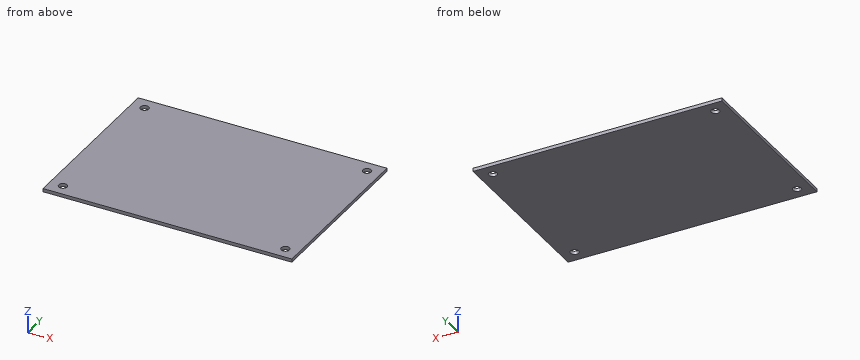
from build123d import *

# Parameters (mm, degrees)
SKETCH1_W           = 155
SKETCH1_H           = 110
BOSS_EXTRUDE1_DEPTH = 80
SKETCH2_W           = 151
SKETCH2_H           = 106
CUT_EXTRUDE1_DEPTH  = 78
SKETCH3_R           = 2.5
CUT_EXTRUDE2_DEPTH  = 2
SKETCH7_R           = 1.6
CUT_EXTRUDE7_DEPTH  = 2
SKETCH4_W           = 27.5
SKETCH4_H           = 46.8
CUT_EXTRUDE8_DEPTH  = 2
SKETCH8_W           = 4
SKETCH8_H           = 53
CUT_EXTRUDE9_DEPTH  = 2
SKETCH9_W           = 14
SKETCH9_H           = 14
CUT_EXTRUDE10_DEPTH = 2
SKETCH10_W          = 25.2
SKETCH10_H          = 71.2
SKETCH10_R          = 1.25
CUT_EXTRUDE12_DEPTH = 2
SKETCH11_R          = 2.5
SKETCH11_R_2        = 4.5
CUT_EXTRUDE13_DEPTH = 2
SKETCH12_W          = 151
SKETCH12_H          = 2
CUT_EXTRUDE14_DEPTH = 80


with BuildPart() as part:
    # Sketch1 → Boss-Extrude1 (new body)
    with BuildSketch(Plane.XY):
        with Locations((77.5, 55)):
            Rectangle(SKETCH1_W, SKETCH1_H)
    extrude(amount=BOSS_EXTRUDE1_DEPTH)

    # Sketch2 → Cut-Extrude1 (cut)
    with BuildSketch(Plane.XY.offset(80)):
        with Locations((77.5, 55)):
            Rectangle(SKETCH2_W, SKETCH2_H)
    extrude(amount=-CUT_EXTRUDE1_DEPTH, mode=Mode.SUBTRACT)

    # Sketch3 → Cut-Extrude2 (cut)
    with BuildSketch(Plane.XY.offset(2)):
        with Locations((145, 100.5)):
            Circle(SKETCH3_R)
        with Locations((145, 9.5)):
            Circle(SKETCH3_R)
        with Locations((10, 9.5)):
            Circle(SKETCH3_R)
        with Locations((10, 100.5)):
            Circle(SKETCH3_R)
    extrude(amount=-CUT_EXTRUDE2_DEPTH, mode=Mode.SUBTRACT)

    # Sketch7 → Cut-Extrude7 (cut)
    with BuildSketch(Plane(origin=(0, 110, 0), x_dir=(1, 0, 0), z_dir=(0, 1, 0))):
        with Locations((44.48, -20.14450396)):
            Circle(SKETCH7_R)
        with Locations((95.28, -17.14)):
            Circle(SKETCH7_R)
        with Locations((95.28, -62.86)):
            Circle(SKETCH7_R)
        with Locations((44.48, -47.62)):
            Circle(SKETCH7_R)
    extrude(amount=-CUT_EXTRUDE7_DEPTH, mode=Mode.SUBTRACT)

    # Sketch4 → Cut-Extrude8 (cut)
    with BuildSketch(Plane(origin=(155, 0, 0), x_dir=(0, 0, -1), z_dir=(1, 0, 0))):
        with Locations((-40, 82.5)):
            Rectangle(SKETCH4_W, SKETCH4_H)
    extrude(amount=-CUT_EXTRUDE8_DEPTH, mode=Mode.SUBTRACT)

    # Sketch8 → Cut-Extrude9 (cut)
    with BuildSketch(Plane(origin=(155, 0, 0), x_dir=(0, 0, -1), z_dir=(1, 0, 0))):
        with Locations((-68, 28.5)):
            Rectangle(SKETCH8_W, SKETCH8_H)
        with Locations((-76, 28.5)):
            Rectangle(SKETCH8_W, SKETCH8_H)
        with Locations((-60, 28.5)):
            Rectangle(SKETCH8_W, SKETCH8_H)
        with Locations((-52, 28.5)):
            Rectangle(SKETCH8_W, SKETCH8_H)
        with Locations((-44, 28.5)):
            Rectangle(SKETCH8_W, SKETCH8_H)
        with Locations((-36, 28.5)):
            Rectangle(SKETCH8_W, SKETCH8_H)
        with Locations((-28, 28.5)):
            Rectangle(SKETCH8_W, SKETCH8_H)
        with Locations((-20, 28.5)):
            Rectangle(SKETCH8_W, SKETCH8_H)
        with Locations((-12, 28.5)):
            Rectangle(SKETCH8_W, SKETCH8_H)
        with Locations((-4, 28.5)):
            Rectangle(SKETCH8_W, SKETCH8_H)
    extrude(amount=-CUT_EXTRUDE9_DEPTH, mode=Mode.SUBTRACT)

    # Sketch9 → Cut-Extrude10 (cut)
    with BuildSketch(Plane(origin=(0, 110, 0), x_dir=(1, 0, 0), z_dir=(0, 1, 0))):
        with Locations((120, -19)):
            Rectangle(SKETCH9_W, SKETCH9_H)
    extrude(amount=-CUT_EXTRUDE10_DEPTH, mode=Mode.SUBTRACT)

    # Sketch10 → Cut-Extrude12 (cut)
    with BuildSketch(Plane.ZY):
        with Locations((58, 55)):
            Rectangle(SKETCH10_W, SKETCH10_H)
        with Locations((42.5, 92.5)):
            Circle(SKETCH10_R)
        with Locations((73.5, 92.5)):
            Circle(SKETCH10_R)
        with Locations((42.5, 17.5)):
            Circle(SKETCH10_R)
        with Locations((73.5, 17.5)):
            Circle(SKETCH10_R)
    extrude(amount=-CUT_EXTRUDE12_DEPTH, mode=Mode.SUBTRACT)

    # Sketch11 → Cut-Extrude13 (cut)
    with BuildSketch(Plane.ZY):
        with Locations((20, 55)):
            Circle(SKETCH11_R)
        with Locations((20, 40)):
            Circle(SKETCH11_R)
        with Locations((20, 25)):
            Circle(SKETCH11_R)
        with Locations((20, 82.5)):
            Circle(SKETCH11_R_2)
    extrude(amount=-CUT_EXTRUDE13_DEPTH, mode=Mode.SUBTRACT)

    # Sketch12 → Cut-Extrude14 (cut)
    with BuildSketch(Plane.XY.offset(80)):
        Polygon((0, 110), (0, 108), (2, 108), (153, 108), (155, 108), (155, 110), align=None)
        Polygon((2, 108), (0, 108), (0, 0), (2, 0), (2, 2), align=None)
        Polygon((155, 108), (153, 108), (153, 2), (153, 0), (155, 0), align=None)
        with Locations((77.5, 1)):
            Rectangle(SKETCH12_W, SKETCH12_H)
    extrude(amount=-CUT_EXTRUDE14_DEPTH, mode=Mode.SUBTRACT)


solid = part.part
For this review, take the finished solid that the model builds, in its own axes (mm). Give positions to 0.01 mm unless a question says otherwise; leave off trailing zeros. Loops run counter-clockwise (first coordinate to the right, second up) from the corner with the lowest first, then second, coordinate; pieces in that order, holes last. Notation, with made-up numbers: (-3.5, -14.5) -> (24.5, -14.5) arc R12 ccw to (24.5, -10.5) -> close; hole circle Ø5 at (-38, -30). An arc over 180 degrees is marked (long way). One line per question, with ' | ' between items.
1) We need section B-B (y = 9.5). Write out the cut boundary in (x, z).
Resolved:
outline: (2, 0) -> (7.5, 0) -> (7.5, 2) -> (2, 2) -> close; (12.5, 0) -> (142.5, 0) -> (142.5, 2) -> (12.5, 2) -> close; (147.5, 0) -> (153, 0) -> (153, 2) -> (147.5, 2) -> close
2) We need section A-A (x = 10). Write out the cut boundary in (y, z), plus the area to 3 significant figures.
Resolved:
outline: (2, 0) -> (7, 0) -> (7, 2) -> (2, 2) -> close; (12, 0) -> (98, 0) -> (98, 2) -> (12, 2) -> close; (103, 0) -> (108, 0) -> (108, 2) -> (103, 2) -> close | area: 192 mm2
3) To check wall thickness, follow probe 1 along Y at (x, z) = (145, 0.55); probe 2 along X at (y, z) = (99, 1.6). State the ranges of each line that lie inside material, in increasing order.
Resolved:
probe 1: y = 2 to 7, 12 to 98, 103 to 108 | probe 2: x = 2 to 8, 12 to 143, 147 to 153
